Design review of the part built by this model. Coordinates are the model's own, in mm. Give positions to 0.01 mm unless a question says otherwise; leave off trailing zeros. Write each loop counter-clockwise with the first axis right and the second up, starting at its lowest first coordinate (ties: lowest second). Pieces come first, ordered by that corner, then holes. Notation, with made-up numbers: M 5,19.5 L 61,19.5 A23 ccw 61,32.5 Z; hole C -34,60 d4. An arc over 180 degrees is marked long. Write each question's results on one line, items separated by ' | '. Start each with the question number.
from build123d import *
from build123d.topology import SkipClean

# Parameters (mm, degrees)
SKETCH1_R               = 2.5
SKETCH1_R_2             = 3.025
BOSS_EXTRUDE1_DEPTH     = 10
BOSS_EXTRUDE2_START     = 10
SKETCH1_3_R             = 2.5
SKETCH1_3_R_2           = 3.025
BOSS_EXTRUDE2_DEPTH     = 30
CUT_EXTRUDE1_DEPTH      = 261.765043932
CUT_EXTRUDE1_DEPTH_BACK = 261.765043932


with BuildPart() as part:
    # Sketch1 → Boss-Extrude1 (new body)
    with BuildSketch(Plane(origin=(0, 0, 0), x_dir=(1, 0, 0), z_dir=(0, 1, 0))):
        with BuildLine():
            Line((90.176952733, -149.337855292), (102.16592726, 130.147858994))
            ThreePointArc((102.16592726, 130.147858994), (0.259643783, 236.519287565), (-101.646639695, 130.147858994))
            Line((-101.646639695, 130.147858994), (-89.657665168, -149.337855292))
            ThreePointArc((-89.657665168, -149.337855292), (0.259643783, -235.480712435), (90.176952733, -149.337855292))
        make_face()
        with Locations(Location((95.172358786, 130.447858994, 0), (0, 0, 270))):
            Circle(SKETCH1_R, mode=Mode.SUBTRACT)
        with Locations(Location((90.029501643, 10.558113726, 0), (0, 0, 270))):
            Circle(SKETCH1_R, mode=Mode.SUBTRACT)
        with Locations(Location((-94.653071221, 130.447858994, 0), (0, 0, 270))):
            Circle(SKETCH1_R_2, mode=Mode.SUBTRACT)
        with Locations(Location((-89.510214078, 10.558113726, 0), (0, 0, 270))):
            Circle(SKETCH1_R, mode=Mode.SUBTRACT)
        with Locations(Location((84.886644501, -109.331631542, 0), (0, 0, 270))):
            Circle(SKETCH1_R_2, mode=Mode.SUBTRACT)
        with Locations(Location((0.259643783, -228.480712435, 0), (0, 0, 270))):
            Circle(SKETCH1_R, mode=Mode.SUBTRACT)
        with Locations(Location((-84.367356936, -109.331631542, 0), (0, 0, 270))):
            Circle(SKETCH1_R, mode=Mode.SUBTRACT)
        with Locations(Location((0.259643783, 229.519287565, 0), (0, 0, 270))):
            Circle(SKETCH1_R, mode=Mode.SUBTRACT)
        with BuildLine():
            Line((-93.159737328, 118.968749538), (-89.00538555, 22.122937467))
            ThreePointArc((-89.00538555, 22.122937467), (-88.169117034, 19.562052023), (-86.125454336, 17.806796467))
            ThreePointArc((-86.125454336, 17.806796467), (-81.517564394, 10.900970869), (-85.517143342, 3.625914501))
            ThreePointArc((-85.517143342, 3.625914501), (-87.402986464, 1.702096679), (-88.016880185, -0.920995729))
            Line((-88.016880185, -0.920995729), (-87.181946752, -20.384876194))
            Line((-87.181946752, -20.384876194), (-86.67600341, -32.179374194))
            Line((-86.67600341, -32.179374194), (-83.862528408, -97.766807801))
            ThreePointArc((-83.862528408, -97.766807801), (-83.026259891, -100.327693245), (-80.982597194, -102.082948801))
            ThreePointArc((-80.982597194, -102.082948801), (-76.374707251, -108.988774399), (-80.3742862, -116.263830767))
            ThreePointArc((-80.3742862, -116.263830767), (-82.260129321, -118.187648589), (-82.874023042, -120.810740997))
            Line((-82.874023042, -120.810740997), (-81.665015484, -148.994998149))
            ThreePointArc((-81.665015484, -148.994998149), (-60.590195056, -200.447039521), (-11.53874162, -226.627481329))
            ThreePointArc((-11.53874162, -226.627481329), (-8.699029781, -226.207678989), (-6.55818493, -224.295355623))
            ThreePointArc((-6.55818493, -224.295355623), (0.259643783, -220.480712435), (7.077472495, -224.295355623))
            ThreePointArc((7.077472495, -224.295355623), (9.218317346, -226.207678989), (12.058029185, -226.627481329))
            ThreePointArc((12.058029185, -226.627481329), (61.109482621, -200.447039521), (82.184303049, -148.994998149))
            Line((82.184303049, -148.994998149), (83.393310607, -120.810740997))
            ThreePointArc((83.393310607, -120.810740997), (82.779416886, -118.187648589), (80.893573765, -116.263830767))
            ThreePointArc((80.893573765, -116.263830767), (76.893994816, -108.988774399), (81.501884759, -102.082948801))
            ThreePointArc((81.501884759, -102.082948801), (83.545547456, -100.327693245), (84.381815973, -97.766807801))
            Line((84.381815973, -97.766807801), (88.53616775, -0.920995729))
            ThreePointArc((88.53616775, -0.920995729), (87.922274029, 1.702096679), (86.036430907, 3.625914501))
            ThreePointArc((86.036430907, 3.625914501), (82.036851959, 10.900970869), (86.644741901, 17.806796467))
            ThreePointArc((86.644741901, 17.806796467), (88.688404599, 19.562052023), (89.524673116, 22.122937467))
            Line((89.524673116, 22.122937467), (93.679024893, 118.968749538))
            ThreePointArc((93.679024893, 118.968749538), (93.065131171, 121.591841947), (91.17928805, 123.515659768))
            ThreePointArc((91.17928805, 123.515659768), (87.172935393, 130.543907811), (91.346884611, 137.473935234))
            ThreePointArc((91.346884611, 137.473935234), (93.356308479, 139.491004193), (93.938902548, 142.277926441))
            ThreePointArc((93.938902548, 142.277926441), (68.13705429, 199.547413348), (12.025979479, 227.779961722))
            ThreePointArc((12.025979479, 227.779961722), (9.216649508, 227.31734246), (7.115315645, 225.396210642))
            ThreePointArc((7.115315645, 225.396210642), (0.259643783, 221.519287565), (-6.59602808, 225.396210642))
            ThreePointArc((-6.59602808, 225.396210642), (-8.697361943, 227.31734246), (-11.506691914, 227.779961722))
            ThreePointArc((-11.506691914, 227.779961722), (-67.617766725, 199.547413348), (-93.419614983, 142.277926441))
            ThreePointArc((-93.419614983, 142.277926441), (-92.837020914, 139.491004193), (-90.827597046, 137.473935234))
            ThreePointArc((-90.827597046, 137.473935234), (-86.653647828, 130.543907811), (-90.660000485, 123.515659768))
            ThreePointArc((-90.660000485, 123.515659768), (-92.545843606, 121.591841947), (-93.159737328, 118.968749538))
        make_face(mode=Mode.SUBTRACT)
    extrude(amount=BOSS_EXTRUDE1_DEPTH)

    # Sketch1_3 → Boss-Extrude2 (add)
    with BuildSketch(Plane(origin=(0, 0, 0), x_dir=(1, 0, 0), z_dir=(0, 1, 0)).offset(BOSS_EXTRUDE2_START)):
        with BuildLine():
            Line((90.176952733, -149.337855292), (102.16592726, 130.147858994))
            ThreePointArc((102.16592726, 130.147858994), (0.259643783, 236.519287565), (-101.646639695, 130.147858994))
            Line((-101.646639695, 130.147858994), (-89.657665168, -149.337855292))
            ThreePointArc((-89.657665168, -149.337855292), (0.259643783, -235.480712435), (90.176952733, -149.337855292))
        make_face()
        with Locations(Location((95.172358786, 130.447858994, 0), (0, 0, 270))):
            Circle(SKETCH1_3_R, mode=Mode.SUBTRACT)
        with Locations(Location((90.029501643, 10.558113726, 0), (0, 0, 270))):
            Circle(SKETCH1_3_R, mode=Mode.SUBTRACT)
        with Locations(Location((-94.653071221, 130.447858994, 0), (0, 0, 270))):
            Circle(SKETCH1_3_R_2, mode=Mode.SUBTRACT)
        with Locations(Location((-89.510214078, 10.558113726, 0), (0, 0, 270))):
            Circle(SKETCH1_3_R, mode=Mode.SUBTRACT)
        with Locations(Location((84.886644501, -109.331631542, 0), (0, 0, 270))):
            Circle(SKETCH1_3_R_2, mode=Mode.SUBTRACT)
        with Locations(Location((0.259643783, -228.480712435, 0), (0, 0, 270))):
            Circle(SKETCH1_3_R, mode=Mode.SUBTRACT)
        with Locations(Location((-84.367356936, -109.331631542, 0), (0, 0, 270))):
            Circle(SKETCH1_3_R, mode=Mode.SUBTRACT)
        with Locations(Location((0.259643783, 229.519287565, 0), (0, 0, 270))):
            Circle(SKETCH1_3_R, mode=Mode.SUBTRACT)
    extrude(amount=BOSS_EXTRUDE2_DEPTH)

    # Sketch2 → Cut-Extrude1 (cut, two sides: drawn at the far end of the back side and taken through both)
    with SkipClean():  # the faces are left unmerged after this step: merging them gives an invalid solid
        with BuildSketch(Plane.XY.offset(-CUT_EXTRUDE1_DEPTH_BACK)):
            with BuildLine():
                Line((-101.646639695, 40), (-101.646639695, 25))
                ThreePointArc((-101.646639695, 25), (-51.242517852, 36.229905144), (0.259643782, 40))
                Line((0.259643782, 40), (-101.646639695, 40))
            make_face()
            with BuildLine():
                Line((102.16592726, 40), (0.259643782, 40))
                ThreePointArc((0.259643782, 40), (51.761805417, 36.229905144), (102.16592726, 25))
                Line((102.16592726, 25), (102.16592726, 40))
            make_face()
        extrude(amount=CUT_EXTRUDE1_DEPTH + CUT_EXTRUDE1_DEPTH_BACK, mode=Mode.SUBTRACT)


solid = part.part
Q1. The part is to be moulded in two halves that separate along X. For faces 1 (the flat face through (-91, 0, -2)), 2 (the flat face through (96.088, 13.991, 11.551)), 3 (the cylindrical face through (60.574, 4.93, 201.034)), say which applies: pulls with the +X half, pulls with the -X half, needs draft (parallel to the pull), parting line crosses it, or undercut.
Q2. For pin 1 Ø3 at (x, z) = (90.03, -10.56) entering from +Y; pin 2 Ø1.5 at (x, z) = (57.5, -108) entering from -Y; pin 3 Ø3 at (y, z) = (25, -114) entering from -X; pin 4 Ø3 at (y, z) = (5.5, -6) entering from -X, all flat-tipped, find the tip position at first contact; note any pin that passes through.
Q3. We need section A-A on z = -79. Write out the cut boundary in (x, y), and give its area (3 significant figures).
Q4. We need section D-D on x = 23.5. Write out the cut boundary in (y, z).
Q5. Wall thickness on line 1 along X through (y, z) = (7, 185); line 2 along Z through (x, y) = (-0.5, 21.5); line 3 along Z through (x, y) = (-82.5, 24.5): over which ranges is each line inside the solid? List them lowest first. Write a range as from..to.
Q6. We need section C-C on z = 161. Write out the cut boundary in (x, y), and give its area (3 significant figures).
Q7. We need section B-B on x = -53.5. Write out the cut boundary in (y, z).
Answer sheet:
1) face 1: needs draft | face 2: pulls with the +X half | face 3: undercut
2) pin 1: through | pin 2: y = 10 | pin 3: x = -101.02 | pin 4: x = -96.39
3) outline: M -99.45,0 L -91.45,0 L -91.45,10 L 91.96,10 L 91.96,0 L 99.97,0 L 99.97,25.65 A353.66 ccw -99.45,25.65 Z | area: 5,200 mm^2
4) outline: M 0,-233.84 L 39.24,-233.84 L 39.24,232.43 L 0,232.43 L 0,224.12 L 10,224.12 L 10,-225.6 L 0,-225.6 Z
5) line 1: -80.6..-71.59, 72.11..81.12 | line 2: -236.52..-231.9, -227.14..226.1, 230.86..235.48 | line 3: -194.14..107.67, 110.99..180.85
6) outline: M -88.39,0 L -80.26,0 L -80.26,10 L 80.78,10 L 80.78,0 L 88.91,0 L 88.91,28.71 A353.66 ccw -88.39,28.71 Z | area: 4,820 mm^2
7) outline: M 0,-221.2 L 35.89,-221.2 L 35.89,217.66 L 0,217.66 L 0,207.4 L 10,207.4 L 10,-211.63 L 0,-211.63 Z
